The listing builds one solid part. Answer for the finished solid, in the listing's coordinates (mm). Give positions to 0.01 mm unless a question says otherwise; leave off trailing zeros. Write each loop counter-clockwise with the first axis right and the second up, starting at its lowest first coordinate (ties: lowest second). Pieces come first, ordered by that corner, then holes. Notation, with made-up numbers: (13, 42) - (43, 42) arc R20 ccw to (43, 56) - close; hole circle Ø4 at (78, 32). An arc over 180 degrees is marked (long way). Return JSON: item names as keys, results as strings.
from build123d import *

# Parameters (mm, degrees)
SKETCH_W            = 347
SKETCH_H            = 420
PAD_DEPTH           = 3
SKETCH001_R         = 1.75
POCKET_DEPTH        = 3.001
POCKET001_DEPTH     = 5
SKETCH003_R         = 1.75
POCKET002_DEPTH     = 3.001
SKETCH005_W         = 22.5
SKETCH005_H         = 15
POCKET003_DEPTH     = 3
LINEARPATTERN_COUNT = 2
LINEARPATTERN_PITCH = 58
SKETCH006_R         = 2.1
SKETCH006_R_2       = 2
POCKET004_DEPTH     = 3.001


with BuildPart() as part:
    # Sketch → Pad (new body)
    with BuildSketch(Plane.XZ):
        with Locations((173.5, 210)):
            Rectangle(SKETCH_W, SKETCH_H)
    extrude(amount=PAD_DEPTH)

    # Sketch001 (on Face6 of Pad) → Pocket (cut, through all)
    with BuildSketch(Plane.XZ.offset(3)):
        with Locations((53.5, 45)):
            Circle(SKETCH001_R)
        with Locations((293.5, 45)):
            Circle(SKETCH001_R)
        with Locations((293.5, 410)):
            Circle(SKETCH001_R)
        with Locations((53.5, 410)):
            Circle(SKETCH001_R)
    extrude(amount=-POCKET_DEPTH, mode=Mode.SUBTRACT)

    # Sketch002 (on Face5 of Pocket) → Pocket001 (cut)
    with BuildSketch(Plane.XZ.offset(3)):
        with BuildLine():
            Line((53, 356), (53, 115))
            ThreePointArc((53, 115), (55.928932, 107.928932), (63, 105))
            Line((63, 105), (284, 105))
            ThreePointArc((284, 105), (291.071068, 107.928932), (294, 115))
            Line((294, 115), (294, 356))
            ThreePointArc((294, 356), (291.071068, 363.071068), (284, 366))
            Line((284, 366), (63, 366))
            ThreePointArc((63, 366), (55.928932, 363.071068), (53, 356))
        make_face()
    extrude(amount=-POCKET001_DEPTH, mode=Mode.SUBTRACT)

    # Sketch003 (on Face5 of Pocket001) → Pocket002 (cut, through all)
    with BuildSketch(Plane.XZ.offset(3)):
        with Locations((129.5, 30)):
            Circle(SKETCH003_R)
        with Locations((129.5, 95)):
            Circle(SKETCH003_R)
        with Locations((217.5, 95)):
            Circle(SKETCH003_R)
        with Locations((217.5, 30)):
            Circle(SKETCH003_R)
    extrude(amount=-POCKET002_DEPTH, mode=Mode.SUBTRACT)

    # Sketch005 (on Face5 of Pocket002) → Pocket003 (cut)
    with BuildSketch(Plane.XZ.offset(3)):
        with Locations((158.5, 84.9)):
            Rectangle(SKETCH005_W, SKETCH005_H)
        with Locations((189, 84.9)):
            Rectangle(SKETCH005_W, SKETCH005_H)
    pocket003 = extrude(amount=-POCKET003_DEPTH, mode=Mode.SUBTRACT)

    # LinearPattern: Pocket003 ×2
    with Locations(*[(0, 0, -i * LINEARPATTERN_PITCH) for i in range(1, LINEARPATTERN_COUNT)]):
        add(pocket003, mode=Mode.SUBTRACT)

    # Sketch006 (on Face5 of LinearPattern) → Pocket004 (cut, through all)
    with BuildSketch(Plane.XZ.offset(3)):
        with Locations((40.75, 330.5)):
            Circle(SKETCH006_R)
        with Locations((40.75, 305.5)):
            Circle(SKETCH006_R)
        with Locations((40.75, 165.5)):
            Circle(SKETCH006_R)
        with Locations((40.75, 140.5)):
            Circle(SKETCH006_R)
        with Locations((304, 254.5)):
            Circle(SKETCH006_R_2)
        with Locations((304, 216.5)):
            Circle(SKETCH006_R_2)
    extrude(amount=-POCKET004_DEPTH, mode=Mode.SUBTRACT)


solid = part.part
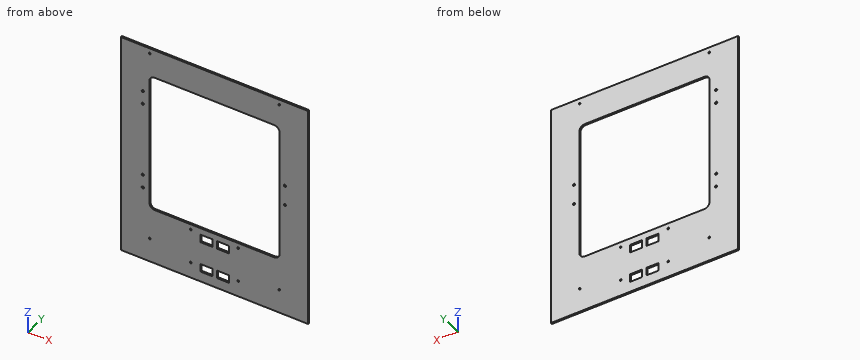
Item 1: A cutting plane is placed at B-B on y = -1.25. Give the number of separate pieces and of enclosed holes in the cut face, then the cut area to 3 significant figures.
Answer below:
{"separate pieces": "1", "enclosed holes": "19", "area": "81,400 mm²"}
Item 2: Consider L1, parallel to X at y = -1.8, z = 330.5; L2, parallel to Z at x = 40.75, y = -0.8; L3, parallel to X at y = -2.3, z = 254.5. Determine where each line is inside the solid, lowest interval first.
Answer below:
{"L1": "x = 0 to 38.65, 42.85 to 53, 294 to 347", "L2": "z = 0 to 138.4, 142.6 to 163.4, 167.6 to 303.4, 307.6 to 328.4, 332.6 to 420", "L3": "x = 0 to 53, 294 to 302, 306 to 347"}
Item 3: A cutting plane is placed at A-A on x = 120. Determine the outline of the cut face in (y, z).
Answer below:
{"outline": "(-3, 0) - (0, 0) - (0, 105) - (-3, 105) - close; (-3, 366) - (0, 366) - (0, 420) - (-3, 420) - close"}
